```python
from build123d import *

# Parameters (mm, degrees)
EXTRUDE_1_DEPTH     = 4
CHAMFER_1_SIZE      = 0.2
CHAMFER_1_SIZE_2    = 0.19070336
CHAMFER_1_SIZE_3    = 0.244096934
SKETCH_2_R          = 2.75
CUT_EXTRUDE_1_DEPTH = 17.881943016
SKETCH_3_R          = 1.5
CUT_EXTRUDE_2_DEPTH = 17.881943152


with BuildPart() as part:
    # 草图1 → 凸台-拉伸1 (new, symmetric)
    with BuildSketch(Plane(origin=(0, 0, 0), x_dir=(1, 0, 0), z_dir=(0, 1, 0))):
        with BuildLine():
            Line((-0.5, -2.958039892), (-0.5, -9.987492178))
            ThreePointArc((-0.5, -9.987492178), (0, 10), (0.5, -9.987492178))
            Line((0.5, -9.987492178), (0.5, -2.958039892))
            ThreePointArc((0.5, -2.958039892), (0, 3), (-0.5, -2.958039892))
        make_face()
    extrude(amount=EXTRUDE_1_DEPTH, both=True)

    # 倒角1
    # the kernel refuses this chamfer: 0.244096934, 0.2, 0.19070336 mm, written as the material it takes off along each edge
    with BuildSketch(Plane(origin=(0, 4, 0), x_dir=(-0.0031415874858795653, 0, 0.9999950652018581), z_dir=(0.9999950652018581, 0, 0.0031415874858795653))) as chamfer_1_piece_1:
        Polygon((10 - CHAMFER_1_SIZE, 0), (10, CHAMFER_1_SIZE), (10, 0), align=None)
    revolve(axis=Axis((0, 4, 0), (0, -1, 0)), revolution_arc=359.64, mode=Mode.SUBTRACT)
    with BuildSketch(Plane(origin=(0, -4, 0), x_dir=(-0.0031415874858795653, 0, 0.9999950652018581), z_dir=(0.9999950652018581, 0, 0.0031415874858795653))) as chamfer_1_piece_2:
        Polygon((10, -CHAMFER_1_SIZE), (10 - CHAMFER_1_SIZE, 0), (10, 0), align=None)
    revolve(axis=Axis((0, -4, 0), (0, -1, 0)), revolution_arc=359.64, mode=Mode.SUBTRACT)
    with BuildSketch(Plane(origin=(-0.5, -4.671168093, 2.958039892), x_dir=(0, 0, 1), z_dir=(0, 1, 0))) as chamfer_1_piece_3:
        with BuildLine():
            Line((CHAMFER_1_SIZE, 0), (-0.054456761, -0.254456761))
            ThreePointArc((-0.054456761, -0.254456761), (-0.025330071, -0.131833133), (0, 0))
            Line((0, 0), (CHAMFER_1_SIZE, 0))
        make_face()
    extrude(amount=9.342336186, mode=Mode.SUBTRACT)
    with BuildSketch(Plane(origin=(-0.5, 4.50932304, 9.987492178), x_dir=(0, 0, -1), z_dir=(0, -1, 0))) as chamfer_1_piece_4:
        with BuildLine():
            Line((CHAMFER_1_SIZE_2 * 1.00000000187, 0), (0.01186065, -0.197693077))
            ThreePointArc((0.01186065, -0.197693077), (0.005608956, -0.101670471), (0, 0))
            Line((0, 0), (CHAMFER_1_SIZE_2 * 1.00000000187, 0))
        make_face()
    extrude(amount=9.01864608, mode=Mode.SUBTRACT)
    with BuildSketch(Plane(origin=(0.5, 4.514336598, 9.987492178), x_dir=(0, 0, -1), z_dir=(0, -1, 0))) as chamfer_1_piece_5:
        with BuildLine():
            Line((CHAMFER_1_SIZE, 0), (0.011239899, 0.188760101))
            ThreePointArc((0.011239899, 0.188760101), (0.005331916, 0.097056531), (0, 0))
            Line((0, 0), (CHAMFER_1_SIZE, 0))
        make_face()
    extrude(amount=9.028673195, mode=Mode.SUBTRACT)
    with BuildSketch(Plane(origin=(0.5, -4.630296565, 2.958039892), x_dir=(0, 0, 1), z_dir=(0, 1, 0))) as chamfer_1_piece_6:
        with BuildLine():
            Line((CHAMFER_1_SIZE_3 * 0.999999998038, 0), (-0.041587873, 0.203070142))
            ThreePointArc((-0.041587873, 0.203070142), (-0.019758938, 0.105396594), (0, 0))
            Line((0, 0), (CHAMFER_1_SIZE_3 * 0.999999998038, 0))
        make_face()
    extrude(amount=9.26059313, mode=Mode.SUBTRACT)

    # 草图2 → 切除-拉伸1 (cut, through all)
    with BuildSketch(Plane(origin=(-3, 0, 0), x_dir=(0, 0, -1), z_dir=(1, 0, 0))):
        with Locations((-5.666452018, 0)):
            Circle(SKETCH_2_R)
    extrude(amount=-CUT_EXTRUDE_1_DEPTH, mode=Mode.SUBTRACT)

    # 草图3 → 切除-拉伸2 (cut, through all)
    with BuildSketch(Plane(origin=(-3, 0, 0), x_dir=(0, 0, -1), z_dir=(1, 0, 0))):
        with Locations(Location((-5.666452018, 0, 0), (0, 0, 180))):
            Circle(SKETCH_3_R)
    extrude(amount=CUT_EXTRUDE_2_DEPTH, mode=Mode.SUBTRACT)


solid = part.part
```
Work out the finished part from the listing and answer in its coordinate system (mm). A direction names the side the tool comes from. Coordinates: 2 decimals unless noted, no trailing zeros. Loops run counter-clockwise (first coordinate to the right, second up) from the corner with the lowest first, then second, coordinate; pieces in that order, holes last.
1) For a pull along Z with two mould halves and no side action, classify faces 1 (the cylindrical face through (6, 0, -8)), 2 (the flat face through (2.3, -4, -2.3)), 3 (the flat face through (-3, -1, 4)), 4 (the cylindrical face through (0, 0, -3)) as +Z half, -Z half, draft (parallel to the pull), parting line (faces both ways), or undercut.
Results:
face 1: parting line
face 2: draft
face 3: undercut
face 4: undercut
2) A flat-ended cylindrical pin translates along its axis: pin 1 (3 mm diameter, centred on y = 0, z = 6.5, fed in from -X). Find the tip coordinate at first contact, or state that the pin passes through.
Results:
pin 1: stops at x = -3
3) Consider probe 1 along X at (y, z) = (1, 0); probe 2 along Z at (x, y) = (2.75, -0.75); probe 3 along X at (y, z) = (-1.5, 2). Determine where each line is inside the solid, lowest interval first.
Results:
probe 1: x = -10 to -3, 3 to 10
probe 2: z = -9.61 to -1.2, 1.2 to 4.37, 6.97 to 9.61
probe 3: x = -9.8 to -2.24, 2.24 to 9.8
4) Section A-A (z = 0) is taken. Give the vertices of the cut face in (x, y).
Results:
outline: (-10, -3.8) - (-9.8, -4) - (-3, -4) - (-3, 4) - (-9.8, 4) - (-10, 3.8) - close; (3, -4) - (9.8, -4) - (10, -3.8) - (10, 3.8) - (9.8, 4) - (3, 4) - close
5) Section C-C (x = 0) is taken. Give the vertices of the cut face in (y, z), plus the area to 3 significant figures.
Results:
outline: (-4, -9.8) - (-3.8, -10) - (3.8, -10) - (4, -9.8) - (4, -3) - (-4, -3) - close
area: 56.0 mm2
6) Section B-B (y = 1) is taken. Give the vertices of the cut face in (x, z), plus the area to 3 significant figures.
Results:
outline: (-9.51, 3.1) arc R10 ccw (long way) to (8.91, 4.55) - (0.5, 4.55) - (0.5, 3.2) - (0.7, 2.92) arc R3 cw (long way) to (-0.75, 2.9) - (-0.5, 3.16) - (-0.5, 4.55) - (-3, 4.55) - (-3, 3.1) - close; (-5.68, 8.23) - (-3, 8.23) - (-3, 6.78) - (-0.5, 6.78) - (-0.5, 9.8) - (-0.7, 9.98) arc R10 ccw to start; (0.5, 6.78) - (7.35, 6.78) arc R10 ccw to (0.69, 9.98) - (0.5, 9.79) - close
area: 230 mm2
7) Section D-D (x = -2.75) is taken. Give the number of separate pieces and of enclosed holes in the cut face, plus the area to 3 significant figures.
Results:
separate pieces: 2
enclosed holes: 1
area: 127 mm2
8) For faces 5 (the cylindrical face through (-5.507, 0.826, 3.043)), 6 (the flat face through (-0.5, 1, 7)), 7 (the flat face through (2.3, 4, -2.3)), determine the directions among +Z, -Z, +X, -X, +Y, -Y from which every point of the face is accessible in a straight line to the end or side of a thin tool.
Results:
face 5: -X
face 6: +Z, +Y, -Y
face 7: +Z, -Z, +X, -X, +Y
